from build123d import *

# Parameters (mm, degrees)
F0_W         = 100
F0_H         = 72
F1_DEPTH     = 8
F2_T         = -2.5
F3_W         = 10
F3_H         = 10
F4_DEPTH     = 78.7
F5_R         = 4.3455844123
F6_R         = 5
F7_T1_DEPTH  = 20.5
F7_T3_DEPTH  = 91.2
F7_T6_ANGLE  = 90
F7_T8_ANGLE  = 90
F7_T10_ANGLE = 90
F8_SIZE      = 5
F9_T1_DEPTH  = 20.5
F9_T4_ANGLE  = 90


# Not quite as in the source:
# - a fillet or chamfer that OpenCascade refuses, or shapes differently, is made with other operations: its cross-section is extruded or revolved along the edge and cut away or added


with BuildPart() as f1:
    # F0 (on Top) → F1 (new body)
    with BuildSketch(Plane.XY):
        Rectangle(F0_W, F0_H)
    extrude(amount=F1_DEPTH)

    # F2
    f2_openings = [f1.faces().sort_by_distance(p)[0] for p in [
        (0, 0, 0),
    ]]
    offset(amount=F2_T, openings=f2_openings)

    # F3 (on face) → F4 (join)
    with BuildSketch(Plane(origin=(0, 0, 5.5), x_dir=(1, 0, 0), z_dir=(0, 0, -1))):
        with Locations((-39.5, -25.5)):
            Rectangle(F3_W, F3_H)
        with Locations((39.5, -25.5)):
            Rectangle(F3_W, F3_H)
        with Locations((39.5, 25.5)):
            Rectangle(F3_W, F3_H)
        with Locations((-39.5, 25.5)):
            Rectangle(F3_W, F3_H)
    extrude(amount=F4_DEPTH)

    # F5
    f5_edges = [f1.edges().sort_by_distance(p)[0] for p in [
        (-50, 0, 8),
        (0, -36, 8),
        (50, 0, 8),
        (0, 36, 8),
    ]]
    fillet(f5_edges, radius=F5_R)

    # F6
    f6_edges = [f1.edges().sort_by_distance(p)[0] for p in [
        (-44.5, -30.5, -33.85),
    ]]
    fillet(f6_edges, radius=F6_R)

    # F7: fillet of radius 5 on 6 edges, made by hand

    # F7_s2 → F7_t1 (cut)
    with BuildSketch(Plane.XY.offset(-12.5)):
        with BuildLine():
            ThreePointArc((-50, -31), (-48.5355339059, -34.5355339059), (-45, -36))
            Line((-45, -36), (-50, -36))
            Line((-50, -36), (-50, -31))
        make_face()
        with BuildLine():
            ThreePointArc((-45, 36), (-48.5355339059, 34.5355339059), (-50, 31))
            Line((-50, 31), (-50, 36))
            Line((-50, 36), (-45, 36))
        make_face()
        with BuildLine():
            ThreePointArc((45, 36), (48.5355339059, 34.5355339059), (50, 31))
            Line((50, 31), (50, 36))
            Line((50, 36), (45, 36))
        make_face()
    extrude(amount=F7_T1_DEPTH, mode=Mode.SUBTRACT)

    # F7_s4 → F7_t3 (cut)
    with BuildSketch(Plane.XY.offset(-85.7)):
        with BuildLine():
            ThreePointArc((39.5, -30.5), (43.0355339059, -29.0355339059), (44.5, -25.5))
            Line((44.5, -25.5), (44.5, -30.5))
            Line((44.5, -30.5), (39.5, -30.5))
        make_face()
        with BuildLine():
            ThreePointArc((44.5, 25.5), (43.0355339059, 29.0355339059), (39.5, 30.5))
            Line((39.5, 30.5), (44.5, 30.5))
            Line((44.5, 30.5), (44.5, 25.5))
        make_face()
        with BuildLine():
            ThreePointArc((-39.5, 30.5), (-43.0355339059, 29.0355339059), (-44.5, 25.5))
            Line((-44.5, 25.5), (-44.5, 30.5))
            Line((-44.5, 30.5), (-39.5, 30.5))
        make_face()
    extrude(amount=F7_T3_DEPTH, mode=Mode.SUBTRACT)

    # F7_s5 → F7_t6 (revolve, cut)
    with BuildSketch(Plane.XZ.offset(-31)):
        with BuildLine():
            ThreePointArc((45.6544155877, 8), (48.7272077939, 6.7272077939), (50, 3.6544155877))
            Line((50, 3.6544155877), (50, 8))
            Line((50, 8), (45.6544155877, 8))
        make_face()
    revolve(axis=Axis((45, 31, 8), (0, 0, 1)), revolution_arc=F7_T6_ANGLE, mode=Mode.SUBTRACT)

    # F7_s7 → F7_t8 (revolve, cut)
    with BuildSketch(Plane.YZ.offset(-45)):
        with BuildLine():
            ThreePointArc((31.6544155877, 8), (34.7272077939, 6.7272077939), (36, 3.6544155877))
            Line((36, 3.6544155877), (36, 8))
            Line((36, 8), (31.6544155877, 8))
        make_face()
    revolve(axis=Axis((-45, 31, 8), (0, 0, 1)), revolution_arc=F7_T8_ANGLE, mode=Mode.SUBTRACT)

    # F7_s9 → F7_t10 (revolve, cut)
    with BuildSketch(Plane.XZ.offset(31)):
        with BuildLine():
            ThreePointArc((-45.6544155877, 8), (-48.7272077939, 6.7272077939), (-50, 3.6544155877))
            Line((-50, 3.6544155877), (-50, 8))
            Line((-50, 8), (-45.6544155877, 8))
        make_face()
    revolve(axis=Axis((-45, -31, 8), (0, 0, 1)), revolution_arc=F7_T10_ANGLE, mode=Mode.SUBTRACT)

    # F8
    f8_edges = [f1.edges().sort_by_distance(p)[0] for p in [
        (-34.5, -20.5, -33.85),
        (-34.5, 20.5, -33.85),
        (34.5, 20.5, -33.85),
        (34.5, -20.5, -33.85),
    ]]
    chamfer(f8_edges, length=F8_SIZE)

    # F9: fillet of radius 5 on 1 edges, made by hand

    # F9_s2 → F9_t1 (cut)
    with BuildSketch(Plane.XY.offset(-12.5)):
        with BuildLine():
            ThreePointArc((50, -31), (48.5355339059, -34.5355339059), (45, -36))
            Line((45, -36), (50, -36))
            Line((50, -36), (50, -31))
        make_face()
    extrude(amount=F9_T1_DEPTH, mode=Mode.SUBTRACT)

    # F9_s3 → F9_t4 (revolve, cut)
    with BuildSketch(Plane.YZ.offset(45)):
        with BuildLine():
            ThreePointArc((-31.6544155877, 8), (-34.7272077939, 6.7272077939), (-36, 3.6544155877))
            Line((-36, 3.6544155877), (-36, 8))
            Line((-36, 8), (-31.6544155877, 8))
        make_face()
    revolve(axis=Axis((45, -31, 8), (0, 0, 1)), revolution_arc=F9_T4_ANGLE, mode=Mode.SUBTRACT)


solid = f1.part
Here's how the part is built. I have some questions about the finished solid (model axes, mm). A direction names the side the tool comes from. Coordinates: 2 decimals unless noted, no trailing zeros. Loops run counter-clockwise (first coordinate to the right, second up) from the corner with the lowest first, then second, coordinate; pieces in that order, holes last.
1. If we mould it in two halves opening along X, with no side actions, what happens to faces 3 (the flat face through (39, -26, -73.2)), 4 (the flat face through (47.5, 0, 3))? For each: pulls with the +X half, pulls with the -X half, needs draft (parallel to the pull), parting line crosses it, or undercut.
2. I need wall thicknesses on L1, parallel to Y at x = 35.5, z = 3.5; L2, parallel to Z at x = 1, y = 27.5; L3, parallel to X at y = -19.5, z = 4. Which ranges of each line are inside material? Lowest first, please.
3. For P1, Ø5.5, axis at y = 27.5, z = -53.5, coming from the +X side; P2, Ø2.5, axis at y = 28, z = -29, coming from the -X side; P3, Ø1.5, axis at x = -42.5, z = -27, coming from the -Y side, each with a flat end and sliding along its axis, tell me the tip position at first contact or that it passes through.
4. Imagine slicing it at D-D, the plane y = 10. Please give me the cut outline in (x, z).
5. Imagine slicing it at B-B, the plane y = 22. Please give me the cut outline in (x, z).
6. Imagine slicing it at A-A, the plane z = -42. Please give me the cut outline in (x, y).
7. For faces 1 (the flat face through (-40, -26, -73.2)), 2 (the flat face through (-1, 33.5, 3)), which set-ups out of +Z, -Z, +X, -X, +Y, -Y let a thin tool reach every point of the face, with its end or its side?
8. Imagine slicing it at C-C, the plane x = 19. Please give me the cut outline in (y, z).
Taken from the geometry:
1. face 3: needs draft
1. face 4: undercut
2. L1: y = -36 to -33.5, -30.5 to -24.5, 24.5 to 30.5, 33.5 to 36
2. L2: z = 5.5 to 8
2. L3: x = -49.99 to -47.5, 47.5 to 49.99
3. P1: stops at x = 44.5
3. P2: stops at x = -44.34
3. P3: stops at y = -29.97
4. outline: (-50, 0) - (-47.5, 0) - (-47.5, 5.5) - (47.5, 5.5) - (47.5, 0) - (50, 0) - (50, 3.65) arc R4.35 ccw to (45.65, 8) - (-45.65, 8) arc R4.35 ccw to (-50, 3.65) - close
5. outline: (-50, 0) - (-47.5, 0) - (-47.5, 5.5) - (-44.5, 5.5) - (-44.5, -73.2) - (-38, -73.2) - (-38, 5.5) - (38, 5.5) - (38, -73.2) - (44.5, -73.2) - (44.5, 5.5) - (47.5, 5.5) - (47.5, 0) - (50, 0) - (50, 3.65) arc R4.35 ccw to (45.65, 8) - (-45.65, 8) arc R4.35 ccw to (-50, 3.65) - close
6. outline: (-44.5, -25.5) arc R5 ccw to (-39.5, -30.5) - (-34.5, -30.5) - (-34.5, -25.5) - (-39.5, -20.5) - (-44.5, -20.5) - close; (-44.5, 20.5) - (-39.5, 20.5) - (-34.5, 25.5) - (-34.5, 30.5) - (-39.5, 30.5) arc R5 ccw to (-44.5, 25.5) - close; (34.5, -30.5) - (39.5, -30.5) arc R5 ccw to (44.5, -25.5) - (44.5, -20.5) - (39.5, -20.5) - (34.5, -25.5) - close; (34.5, 25.5) - (39.5, 20.5) - (44.5, 20.5) - (44.5, 25.5) arc R5 ccw to (39.5, 30.5) - (34.5, 30.5) - close
7. face 1: -Z, +X, -X, +Y, -Y
7. face 2: -Z
8. outline: (-36, 0) - (-33.5, 0) - (-33.5, 5.5) - (33.5, 5.5) - (33.5, 0) - (36, 0) - (36, 3.65) arc R4.35 ccw to (31.65, 8) - (-31.65, 8) arc R4.35 ccw to (-36, 3.65) - close
